Verification items for the finished model (mm, model axes). A direction names the side the tool comes from. Coordinates: 2 decimals unless noted, no trailing zeros. Order: outer loops, then holes, each group sorted by start corner. A loop starts at its lowest first (then second) coordinate and runs counter-clockwise, first axis right, second up. Notation, with made-up numbers: M -7,71.25 L 49,71.25 A27 ccw 49,94.25 Z; hole C 82,6 d6. An arc over 180 degrees is marked long. Write item = value, one per line.
```python
from build123d import *

# Parameters (mm, degrees)
F1_W = 10
F1_H = 2.5


with BuildPart() as f2:
    # F2: sweep along a path in F0
    with BuildLine(Plane.XZ) as f2_path:
        Line((0, 0), (7.5, 0))
        ThreePointArc((7.5, 0), (9.267767, -0.732233), (10, -2.5))
        Line((10, -2.5), (10, -10))
    # F1 (on Right) → F2 (sweep)
    with BuildSketch(Plane.YZ):
        Rectangle(F1_W, F1_H)
    sweep(path=f2_path.line)


solid = f2.part
```
Item 1: Tool access check on faces 1 (the flat face through (4, 0, -1.25)), 2 (the flat face through (9, 5, -3)). Record the directions out of +Z, -Z, +X, -X, +Y, -Y that give a thin tool (end or side, any length) a straight path to the whole face; none if there is none.
Report:
face_1 = -Z, -X, +Y, -Y
face_2 = +Z, -Z, +X, -X, +Y
Item 2: Sectioned sample at A-A, the plane y = -0.75. Enter the section's corners in (x, z), then the cut area to 3 significant figures.
Report:
outline = M 0,-1.25 L 7.5,-1.25 A1.25 cw 8.75,-2.5 L 8.75,-10 L 11.25,-10 L 11.25,-2.5 A3.75 ccw 7.5,1.25 L 0,1.25 Z
area = 47.3 mm^2
Item 3: Sectioned sample at B-B, the plane z = -7.5. Enter the section's corners in (x, y), then the cut area to 3 significant figures.
Report:
outline = M 8.75,-5 L 11.25,-5 L 11.25,5 L 8.75,5 Z
area = 25.0 mm^2
Item 4: Scan lines: L1, parallel to X at y = -4.5, z = -7.75; L2, parallel to Z at x = 1, y = -1. Record each from-to range of solid material in increasing order. Write a range as from..to.
Report:
L1 = 8.75..11.25
L2 = -1.25..1.25
Item 5: Gauge pin test, flat ends, axial feed: pin 1 (5 mm diameter, centred on y = 0.5, z = -6, fed in from -X); pin 2 (4 mm diameter, centred on x = 3.5, y = 2.5, fed in from -Z); pin 3 (6 mm diameter, centred on y = 2.5, z = -4.5, fed in from -X); pin 4 (3 mm diameter, centred on x = 8.5, y = -1, fed in from +Z). Record the tip position at first contact, or that the pin passes through.
Report:
pin_1 = 8.75
pin_2 = -1.25
pin_3 = 8.25
pin_4 = 1.25
Item 6: Sectioned sample at C-C, the plane x = 10.5. Enter the section's corners in (y, z), then the cut area to 3 significant figures.
Report:
outline = M -5,-10 L 5,-10 L 5,-0.25 L -5,-0.25 Z
area = 97.5 mm^2
